```python
from build123d import *

# Parameters (mm, degrees)
F0_W          = 25.4
F0_H          = 25.4
F1_DEPTH      = 3.175
F1_TAPER      = 3
F3_W          = 5.08
F3_H          = 12.7
F6_DEPTH      = 6.35
F6_DEPTH_BACK = 6.35


with BuildPart() as f1:
    # F0 (on Top) → F1 (new body)
    with BuildSketch(Plane.XY):
        Rectangle(F0_W, F0_H)
    extrude(amount=F1_DEPTH, taper=F1_TAPER)

    # F4: sweep along a path in F2
    with BuildLine(Plane.XZ) as f4_path:
        ThreePointArc((-10.16, 0), (0, -23.5582897328), (10.16, 0))
    # F3 (on face) → F4 (sweep)
    with BuildSketch(Plane(origin=(0, 0, 0), x_dir=(1, 0, 0), z_dir=(0, 0, -1))):
        with Locations((-10.16, 0)):
            Rectangle(F3_W, F3_H)
    sweep(path=f4_path.line)

    # F5 (on Front) → F6 (join, two sides)
    with BuildSketch(Plane.XZ) as f6_sk:
        with BuildLine():
            Line((10.0130578512, -2.535746045), (10.16, 0))
            Line((10.16, 0), (7.62, 0))
            ThreePointArc((7.62, 0), (8.9072265211, -1.1822790439), (10.0130578512, -2.535746045))
        make_face()
    extrude(amount=F6_DEPTH)
    extrude(f6_sk.sketch, amount=-F6_DEPTH_BACK)


solid = f1.part
```
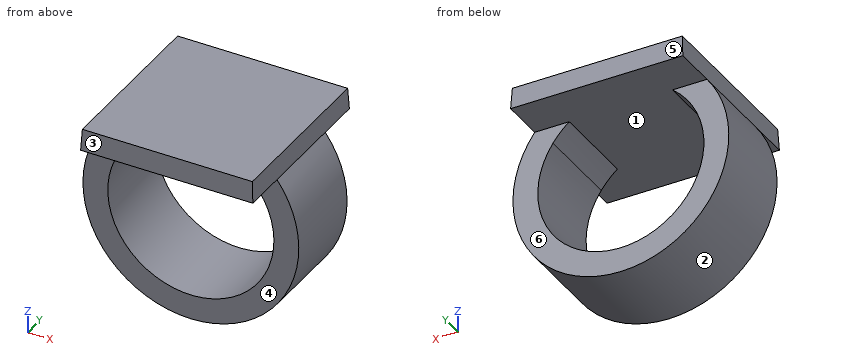
For this review, take the finished solid that the model builds, in its own axes (mm). Face numbers are marked on the shaded views. A direction names the side the tool comes from. Round coordinates to 2 decimals unless told otherwise and drop trailing zeros. Write each loop counter-clockwise with the first axis right and the second up, starting at its lowest first coordinate (ties: lowest second). Pieces come first, ordered by that corner, then holes. Notation, with made-up numbers: (79, 81) -> (101, 81) arc R23 ccw to (101, 104) -> close; hole circle Ø8 at (-19.5, -17.75). An arc over 180 degrees is marked (long way). Use one line per item in the form item = value.
Q1. Clearance check with flat-ended pins moving along their axes: pin 1 Ø5 at (x, y) = (12.5, -10) entering from -Z; pin 2 Ø4 at (y, z) = (-6, -15) entering from -X; pin 3 Ø5 at (x, z) = (3.5, -21) entering from +Y. State where each tip first meets the part, or that it passes through.
Resolved:
pin_1 = 0
pin_2 = -15.54
pin_3 = 6.35
Q2. Consider section C-C (z = -18.25). State the section outline as (x, y) points, then the cut area to 3 significant figures.
Resolved:
outline = (-13.35, -6.35) -> (-8.66, -6.35) -> (-8.66, 6.35) -> (-13.35, 6.35) -> close; (8.66, -6.35) -> (13.35, -6.35) -> (13.35, 6.35) -> (8.66, 6.35) -> close
area = 119 mm²
Q3. The part is to be moulded in two halves that separate along Z. For the marked faces 1, 2, 3 and 4, say which applies: released by +Z, released by -Z, zero draft, split by the parting line, or undercut.
Resolved:
face_1 = undercut
face_2 = split by the parting line
face_3 = released by +Z
face_4 = zero draft
Q4. Machinability: for the marked faces 5 and 6, which of the approach directions +Z, -Z, +X, -X, +Y, -Y give a long, thin tool a straight path to every point of the face, cutting with its end or side? Answer none if there is none.
Resolved:
face_5 = +Z, +X, -X, +Y
face_6 = -Z, +X, -X, +Y
Q5. Consider section A-A (x = 0). State the section outline as (y, z) points (3 decimals), then the cut area to 3 significant figures.
Resolved:
outline = (-12.7, 0) -> (12.7, 0) -> (12.534, 3.175) -> (-12.534, 3.175) -> close; (-6.35, -25.501) -> (6.35, -25.501) -> (6.35, -21.836) -> (-6.35, -21.836) -> close
area = 127 mm²
Q6. Consider section D-D (y = -7.5). State the section outline as (x, z) points (3 decimals), then the cut area to 3 significant figures.
Resolved:
outline = (-12.7, 0) -> (12.7, 0) -> (12.534, 3.175) -> (-12.534, 3.175) -> close
area = 80.1 mm²
Q7. To check wall thickness, follow probe 1 along Z at (x, y) = (0, 2.5) (3 decimals); probe 2 along Z at (x, y) = (3.5, 9.25) (3 decimals); probe 3 along Y at (x, z) = (5, -23). State the ranges of each line that lie inside material, in increasing order. Write a range as from..to.
Resolved:
probe_1 = -25.501..-21.836, 0..3.175
probe_2 = 0..3.175
probe_3 = -6.35..6.35
Q8. Consider section B-B (y = 3.75). State the section outline as (x, z) points (3 decimals), then the cut area to 3 significant figures.
Resolved:
outline = (-12.7, 0) arc R15.913 ccw (long way) to (12.7, 0) -> (12.534, 3.175) -> (-12.534, 3.175) -> close; hole (-7.62, 0) arc R12.247 ccw (long way) to (7.62, 0) -> close
area = 320 mm²
